Read the model definition and answer for the solid it produces. Units are mm, in the model's axes. Face numbers are marked on the shaded views. A direction names the side the tool comes from. Round coordinates to 2 decimals unless told otherwise and drop trailing zeros. Order: outer loops, then holes, each group sorted by start corner. A loop starts at its lowest first (then second) coordinate and runs counter-clockwise, first axis right, second up.
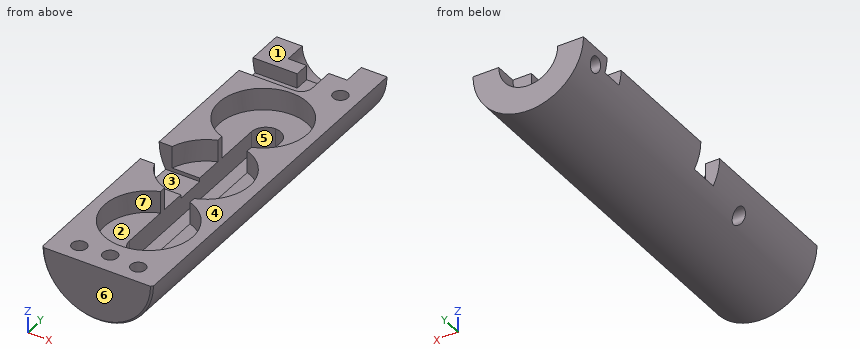
from build123d import *

# Parameters (mm, degrees)
F1_DEPTH  = 50
F2_R      = 6
F3_DEPTH  = 3
F4_R      = 4
F5_DEPTH  = 3
F6_W      = 4
F6_H      = 30
F7_DEPTH  = 6
F8_R      = 1.99999
F9_W      = 9.3910377485
F9_H      = 4
F10_DEPTH = 3.5
F12_D     = 2
F12_DEPTH = 4
F12_TIP   = 0.600860619
F14_DEPTH = 2
F15_R     = 1.5
F16_SIZE  = 0.25
F18_R     = 1
F19_DEPTH = 3
F20_R     = 1
F21_DEPTH = 3


# Not quite as in the source:
# - a fillet or chamfer is up to 0.001 mm smaller than in the source, because OpenCascade refuses the exact size


with BuildPart() as f1:
    # F0 (on Front) → F1 (new body)
    with BuildSketch(Plane.XZ):
        with BuildLine():
            Line((7.5, 0), (-7.5, 0))
            ThreePointArc((-7.5, 0), (0, -7.5), (7.5, 0))
        make_face()
    extrude(amount=F1_DEPTH)

    # F2 (on face) → F3 (cut)
    with BuildSketch(Plane.XY):
        with Locations((0, -39)):
            Circle(F2_R)
        with Locations((0, -26.8)):
            Circle(F2_R)
        with Locations((0, -14.6)):
            Circle(F2_R)
    extrude(amount=-F3_DEPTH, mode=Mode.SUBTRACT)

    # F4 (on face) → F5 (cut)
    with BuildSketch(Plane(origin=(0, 0, 0), x_dir=(-1, 0, 0), z_dir=(0, 1, 0))):
        Circle(F4_R)
    extrude(amount=-F5_DEPTH, mode=Mode.SUBTRACT)

    # F6 (on face) → F7 (cut)
    with BuildSketch(Plane.XY):
        with Locations((0, -27)):
            Rectangle(F6_W, F6_H)
    extrude(amount=-F7_DEPTH, mode=Mode.SUBTRACT)

    # F8 (radius 2 in the source; OpenCascade refuses exactly that, so slightly less here)
    f8_edges = [f1.edges().sort_by_distance(p)[0] for p in [
        (-2, -12, -4.5),
        (2, -12, -4.5),
        (-2, -42, -4.5),
        (2, -42, -4.5),
    ]]
    fillet(f8_edges, radius=F8_R)

    # F9 (on face) → F10 (cut)
    with BuildSketch(Plane.XY):
        with Locations((-4.6955188743, -27)):
            Rectangle(F9_W, F9_H)
    extrude(amount=-F10_DEPTH, mode=Mode.SUBTRACT)

    # F12
    with Locations(Plane.XY):
        with Locations((5, -6), (0, -47.2)):
            Hole(F12_D / 2, depth=F12_DEPTH)
            with Locations((0, 0, -(F12_DEPTH + F12_TIP / 2))):  # 118° drill point
                Cone(0, F12_D / 2, F12_TIP, mode=Mode.SUBTRACT)

    # F13 (on face) → F14 (cut)
    with BuildSketch(Plane.XY):
        Polygon((1.5, -3), (-1.5, -3), (-1.5, -5), (-8.88405554, -5), (-8.88405554, -8), (-1.5, -8), (1.5, -8), align=None)
    extrude(amount=-F14_DEPTH, mode=Mode.SUBTRACT)

    # F15
    f15_edges = [f1.edges().sort_by_distance(p)[0] for p in [
        (1.5, -8, -1),
    ]]
    fillet(f15_edges, radius=F15_R)

    # F16
    f16_edges = [f1.edges().sort_by_distance(p)[0] for p in [
        (0, -50, -7.5),
    ]]
    chamfer(f16_edges, length=F16_SIZE)

    # F18 (on offset) → F19 (cut)
    with BuildSketch(Plane.YZ.offset(-7.5)):
        with Locations((-3, -2)):
            Circle(F18_R)
        with Locations((-35, -4)):
            Circle(F18_R)
    extrude(amount=F19_DEPTH, mode=Mode.SUBTRACT)

    # F20 (on face) → F21 (cut)
    with BuildSketch(Plane.XY):
        with Locations((-4, -47.5)):
            Circle(F20_R)
        with Locations((4, -47.5)):
            Circle(F20_R)
    extrude(amount=-F21_DEPTH, mode=Mode.SUBTRACT)


solid = f1.part
Q1. Flat-ended cylindrical pins translate along their axes: pin 1 (1.5 mm diameter, centred on y = -9.5, z = -3.5, fed in from +X); pin 2 (3 mm diameter, centred on x = 5, y = -6, fed in from -Z); pin 3 (1 mm diameter, centred on y = -10, z = -4, fed in from +X). Find the tip coordinate at first contact, or state that the pin passes through.
Outcome:
pin 1: stops at x = 6.98
pin 2: stops at z = -6.63
pin 3: stops at x = 6.63
Q2. A cutting plane is placed at D-D, the plane y = -26.5. Give the vertices of the cut face in (x, z).
Outcome:
outline: (-6.63, -3.5) arc R7.5 ccw to (7.5, 0) - (5.99, 0) - (5.99, -3) - (2, -3) - (2, -6) - (-2, -6) - (-2, -3.5) - close
Q3. Straight lines are drawn through the part: probe 1 along Y at (x, z) = (0, -2.1); probe 2 along Y at (x, z) = (-4, -1.35); probe 3 along Z at (x, y) = (-6.15, -35). For each, find the intervals that lie inside material, in ascending order.
Outcome:
probe 1: y = -50 to -48.2, -46.2 to -45, -8.6 to -3
probe 2: y = -50 to -48.5, -46.5 to -43.47, -34.53 to -31.27, -22.33 to -19.07, -10.13 to -8, -5 to 0
probe 3: z = -3 to 0
Q4. A cutting plane is placed at C-C, the plane y = -19. Give the vertices of the cut face in (x, z).
Outcome:
outline: (-7.5, 0) arc R7.5 ccw to (7.5, 0) - (4.08, 0) - (4.08, -3) - (2, -3) - (2, -6) - (-2, -6) - (-2, -3) - (-4.08, -3) - (-4.08, 0) - close
Q5. For the marked faces 1, 2 and 3, determine the directions among +Z, -Z, +X, -X, +Y, -Y from which every point of the face is accessible in a straight line to the end or side of a thin tool.
Outcome:
face 1: +Z, +X, -X, +Y, -Y
face 2: +Z
face 3: +Z, -X
Q6. For a pull along Y with two mould halves and no side action, classify the marked faces 4, 5, 6 and 7 as released by +Y, released by -Y, zero draft, split by the parting line, or undercut.
Outcome:
face 4: zero draft
face 5: undercut
face 6: released by -Y
face 7: undercut
Q7. A cutting plane is placed at A-A, the plane y = -39. Give the vertices of the cut face in (x, z).
Outcome:
outline: (-7.5, 0) arc R7.5 ccw to (7.5, 0) - (6, 0) - (6, -3) - (2, -3) - (2, -6) - (-2, -6) - (-2, -3) - (-6, -3) - (-6, 0) - close
Q8. A cutting plane is placed at B-B, the plane y = -10. Give the vertices of the cut face in (x, z).
Outcome:
outline: (-7.5, 0) arc R7.5 ccw to (7.5, 0) - (3.85, 0) - (3.85, -3) - (-3.85, -3) - (-3.85, 0) - close
